from build123d import *

# Parameters (mm, degrees)
SKETCH_1_R      = 7.5
SKETCH_1_R_2    = 4
EXTRUDE_1_DEPTH = 20


with BuildPart() as part:
    # 草图1 → 凸台-拉伸1 (new body)
    with BuildSketch(Plane.XY):
        with BuildLine():
            Line((-25, 10), (25, 10))
            ThreePointArc((25, 10), (35, 0), (25, -10))
            Line((25, -10), (-25, -10))
            ThreePointArc((-25, -10), (-35, 0), (-25, 10))
        make_face()
        Circle(SKETCH_1_R, mode=Mode.SUBTRACT)
        with Locations((-25, 0)):
            Circle(SKETCH_1_R_2, mode=Mode.SUBTRACT)
        with Locations(Location((25, 0, 0), (0, 0, 180))):
            Circle(SKETCH_1_R_2, mode=Mode.SUBTRACT)
    extrude(amount=EXTRUDE_1_DEPTH)


solid = part.part
Read the model definition and answer for the solid it produces. Units are mm, in the model's axes. Give positions to 0.01 mm unless a question says otherwise; leave off trailing zeros. Loops run counter-clockwise (first coordinate to the right, second up) from the corner with the lowest first, then second, coordinate; pieces in that order, holes last. Notation, with made-up numbers: (9, 7) - (23, 7) arc R17 ccw to (23, 16) - close; hole circle Ø6 at (43, 56). An arc over 180 degrees is marked (long way). Answer as CSV lines item,"result". Start each with the question number.
1) Find section B-B (x = 0). Write down the section's boundary in (y, z), then the cut area to 3 significant figures.
2) Straight lines are drawn through the part: L1, parallel to Y at x = 0, z = 13; L2, parallel to Y at x = 25, z = 12.25; L3, parallel to X at y = -3.25, z = 4. For each, find the intervals that lie inside material, in ascending order. Write a range as from..to.
3) Find section C-C (y = 0). Write down the section's boundary in (x, z), then the cut area to 3 significant figures.
4) Find section A-A (z = 13). Write down the section's boundary in (x, y).
5) Find section D-D (y = -4.75). Write down the section's boundary in (x, z).
6) Each of these flat-tipped pins is pushed along its axis until it touches: pin 1 Ø5 at (y, z) = (-8, 7) entering from +X; pin 2 Ø7 at (x, y) = (25, 0) entering from -Z; pin 3 Ø2 at (y, z) = (-7.5, 4) entering from -X; pin 4 Ø1.5 at (y, z) = (2, 10.5) entering from -X. Where does it stop, or does it pass through?
7) Determine the mould class of faces 1 (the face through (-35, 0, 10)), 2 (the face through (35, 0, 10)), 3 (the face through (28.2, 2.4, 9.9)) for opening direction X: released by +X, released by -X, zero draft, split by the parting line, or undercut.
Findings below:
1,outline,"(-10, 0) - (-7.5, 0) - (-7.5, 20) - (-10, 20) - close; (7.5, 0) - (10, 0) - (10, 20) - (7.5, 20) - close"
1,area,"100 mm^2"
2,L1,"-10..-7.5, 7.5..10"
2,L2,"-10..-4, 4..10"
2,L3,"-34.46..-27.33, -22.67..-6.76, 6.76..22.67, 27.33..34.46"
3,outline,"(-35, 0) - (-29, 0) - (-29, 20) - (-35, 20) - close; (-21, 0) - (-7.5, 0) - (-7.5, 20) - (-21, 20) - close; (7.5, 0) - (21, 0) - (21, 20) - (7.5, 20) - close; (29, 0) - (35, 0) - (35, 20) - (29, 20) - close"
3,area,"780 mm^2"
4,outline,"(-25, -10) - (25, -10) arc R10 ccw to (25, 10) - (-25, 10) arc R10 ccw to start; hole circle Ø8 at (-25, 0); hole circle Ø15 at (0, 0); hole circle Ø8 at (25, 0)"
5,outline,"(-33.8, 0) - (-5.8, 0) - (-5.8, 20) - (-33.8, 20) - close; (5.8, 0) - (33.8, 0) - (33.8, 20) - (5.8, 20) - close"
6,pin 1,"x = 33.35"
6,pin 2,"through"
6,pin 3,"x = -32.6"
6,pin 4,"x = -34.92"
7,face 1,"released by -X"
7,face 2,"released by +X"
7,face 3,"undercut"
